Input: dimensioned drawing with shaded views. Units: mm. Origin: part minimum x, y, z. Give positions to 0.01 mm unless a question says otherwise; leave off trailing zeros. Loops run counter-clockwise (first coordinate to the right, second up) from the corner with the lowest first, then second, coordinate; pieces in that order, holes last.
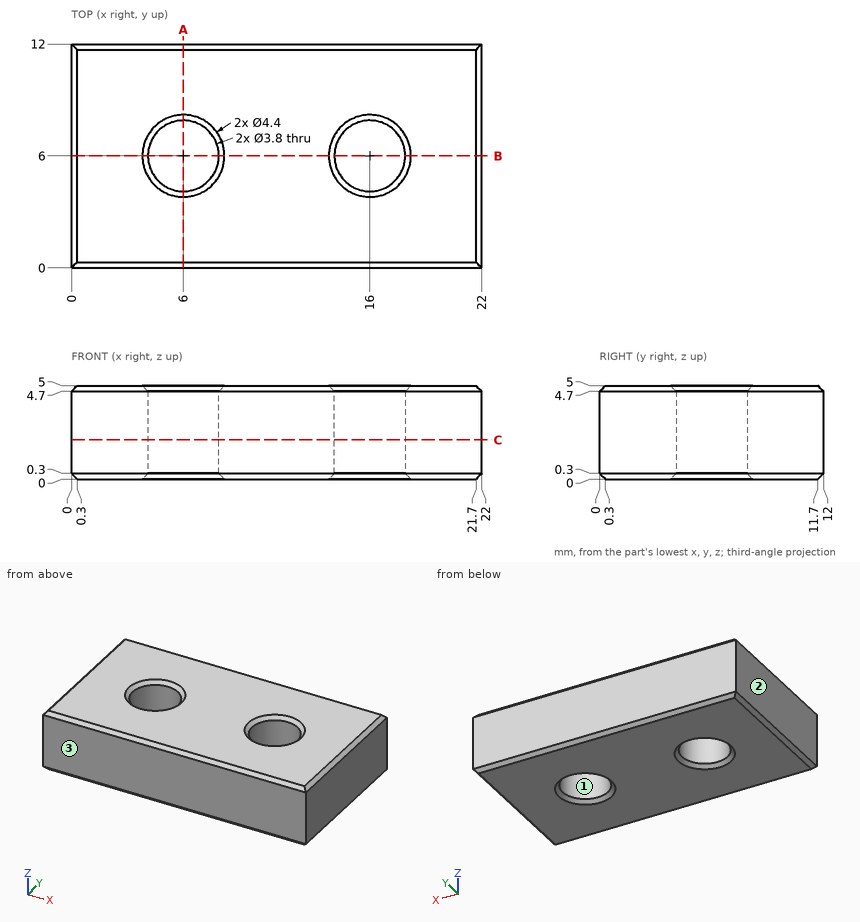
(1) First-contact query: pin 1 (6 mm diameter, centred on x = 6, y = 6, fed in from -Z). Flat tip, straight axial feed; report the tip coordinate or a pass-through.
A:
pin 1: stops at z = 0
(2) Section B-B, the plane y = 6. Return the cut outline in (x, z), then the cut area to 3 significant figures.
A:
outline: (0, 0.3) - (0.3, 0) - (3.8, 0) - (4.1, 0.3) - (4.1, 4.7) - (3.8, 5) - (0.3, 5) - (0, 4.7) - close; (7.9, 0.3) - (8.2, 0) - (13.8, 0) - (14.1, 0.3) - (14.1, 4.7) - (13.8, 5) - (8.2, 5) - (7.9, 4.7) - close; (17.9, 0.3) - (18.2, 0) - (21.7, 0) - (22, 0.3) - (22, 4.7) - (21.7, 5) - (18.2, 5) - (17.9, 4.7) - close
area: 71.5 mm2
(3) Section A-A, the plane x = 6. Return the cut outline in (y, z), then the cut area to 3 significant figures.
A:
outline: (0, 0.3) - (0.3, 0) - (3.8, 0) - (4.1, 0.3) - (4.1, 4.7) - (3.8, 5) - (0.3, 5) - (0, 4.7) - close; (7.9, 0.3) - (8.2, 0) - (11.7, 0) - (12, 0.3) - (12, 4.7) - (11.7, 5) - (8.2, 5) - (7.9, 4.7) - close
area: 40.6 mm2
(4) Mould query, pull axis Y, two halves, no side actions, for the marked faces 1, 2 and 3. Classes: pulls with the +Y half, pulls with the -Y half, needs draft (parallel to the pull), parting line crosses it, or undercut.
A:
face 1: undercut
face 2: needs draft
face 3: pulls with the -Y half
(5) Ray query, line 1 along Y through (x, z) = (16, 2.4); line 2 along X through (y, z) = (6.5, 2.35); line 3 along X through (y, z) = (7.25, 0.6). Return the intervals inside material, ascending.
A:
line 1: y = 0 to 4.1, 7.9 to 12
line 2: x = 0 to 4.17, 7.83 to 14.17, 17.83 to 22
line 3: x = 0 to 4.57, 7.43 to 14.57, 17.43 to 22
(6) Section C-C, the plane z = 2.1. Return the cut outline in (x, y), then the cut area to 3 significant figures.
A:
outline: (0, 0) - (22, 0) - (22, 12) - (0, 12) - close; hole circle Ø3.8 at (6, 6); hole circle Ø3.8 at (16, 6)
area: 241 mm2
